Design review of the part built by this model. Coordinates are the model's own, in mm. A direction names the side the tool comes from. Give positions to 0.01 mm unless a question says otherwise; leave off trailing zeros. Order: outer loops, then holes, each group sorted by start corner. A loop starts at its lowest first (then second) coordinate and runs counter-clockwise, first axis right, second up.
```python
from build123d import *

# Parameters (mm, degrees)
SKETCH1_W           = 83
SKETCH1_H           = 151.45
BOSS_EXTRUDE1_DEPTH = 3
SKETCH2_W           = 83
SKETCH2_H           = 70
BOSS_EXTRUDE2_DEPTH = 3
SKETCH3_W           = 83
SKETCH3_H           = 89
BOSS_EXTRUDE3_DEPTH = 3
SKETCH6_W           = 34
SKETCH6_H           = 28
SKETCH6_R           = 4.15
SKETCH6_H_2         = 30
BOSS_EXTRUDE6_DEPTH = 30
SKETCH7_R           = 16
SKETCH7_R_2         = 15
BOSS_EXTRUDE7_DEPTH = 42
SKETCH8_R           = 5
CUT_EXTRUDE1_DEPTH  = 20.05


with BuildPart() as part:
    # Sketch1 → Boss-Extrude1 (new body)
    with BuildSketch(Plane.XY):
        with Locations((41.5, 75.725)):
            Rectangle(SKETCH1_W, SKETCH1_H)
    extrude(amount=BOSS_EXTRUDE1_DEPTH)

    # Sketch2 → Boss-Extrude2 (add)
    with BuildSketch(Plane(origin=(0, 16.05, 0), x_dir=(-1, 0, 0), z_dir=(0, -1, 0))):
        with Locations((-41.5, -38)):
            Rectangle(SKETCH2_W, SKETCH2_H)
    boss_extrude2 = extrude(amount=-BOSS_EXTRUDE2_DEPTH)

    # Mirror1: Boss-Extrude2 across plane
    add(boss_extrude2.mirror(Plane.ZX.offset(75.725)))

    # Sketch3 → Boss-Extrude3 (add)
    with BuildSketch(Plane(origin=(0, 135.4, 0), x_dir=(1, 0, 0), z_dir=(0, 1, 0))):
        with Locations((41.5, -47.5)):
            Rectangle(SKETCH3_W, SKETCH3_H)
    extrude(amount=-BOSS_EXTRUDE3_DEPTH)

    # Sketch6 → Boss-Extrude6 (add)
    with BuildSketch(Plane(origin=(0, 88.45, 0), x_dir=(1, 0, 0), z_dir=(0, 1, 0))):
        with Locations((21.979, 14)):
            Rectangle(SKETCH6_W, SKETCH6_H)
        with Locations((21.979, 18)):
            Circle(SKETCH6_R, mode=Mode.SUBTRACT)
        with Locations((60.98, 15)):
            Rectangle(SKETCH6_W, SKETCH6_H_2)
        with Locations((60.98, 18)):
            Circle(SKETCH6_R, mode=Mode.SUBTRACT)
    extrude(amount=-BOSS_EXTRUDE6_DEPTH)

    # Sketch7 → Boss-Extrude7 (add)
    with BuildSketch(Plane.XZ.offset(-132.4)):
        with Locations((42, 43)):
            Circle(SKETCH7_R)
        with Locations((42, 43)):
            Circle(SKETCH7_R_2, mode=Mode.SUBTRACT)
    extrude(amount=BOSS_EXTRUDE7_DEPTH)

    # Sketch8 → Cut-Extrude1 (cut, through all)
    with BuildSketch(Plane(origin=(0, 19.05, 0), x_dir=(1, 0, 0), z_dir=(0, 1, 0))):
        with Locations((42, -43)):
            Circle(SKETCH8_R)
    extrude(amount=-CUT_EXTRUDE1_DEPTH, mode=Mode.SUBTRACT)


solid = part.part
```
1. For pin 1 (8.5 mm diameter, centred on y = 79, z = -15.5, fed in from -X); pin 2 (1.5 mm diameter, centred on x = 44, y = 21.5, fed in from +Z); pin 3 (9 mm diameter, centred on x = 63.5, z = -21, fed in from +Y), all flat-tipped, find the tip position at first contact; note any pin that passes through.
Recorded:
pin 1: stops at x = 4.98
pin 2: stops at z = 3
pin 3: stops at y = 88.45
2. Take a section at B-B (y = 94.5). State the section outline as (x, z) points.
Recorded:
outline: (0, 0) - (83, 0) - (83, 3) - (0, 3) - close; circle Ø32 at (42, 43); hole circle Ø30 at (42, 43)
3. For line 1 along Z through (x, y) = (42, 99); line 2 along X through (y, z) = (67, -18); line 3 along Y through (x, z) = (22, 8.5), list the stretches that pass through material, from the lowest coordinate up.
Recorded:
line 1: z = 0 to 3, 27 to 28, 58 to 59
line 2: x = 4.98 to 17.83, 26.13 to 38.98, 43.98 to 56.83, 65.13 to 77.98
line 3: y = 16.05 to 19.05, 132.4 to 135.4
4. Take a section at C-C (x = 42). State the section outline as (y, z) points, then the cut area to 3 significant figures.
Recorded:
outline: (0, 0) - (151.45, 0) - (151.45, 3) - (135.4, 3) - (135.4, 92) - (132.4, 92) - (132.4, 59) - (90.4, 59) - (90.4, 58) - (132.4, 58) - (132.4, 28) - (90.4, 28) - (90.4, 27) - (132.4, 27) - (132.4, 3) - (19.05, 3) - (19.05, 38) - (16.05, 38) - (16.05, 3) - (0, 3) - close; (16.05, 48) - (19.05, 48) - (19.05, 73) - (16.05, 73) - close
area: 985 mm2
5. Take a section at D-D (z = 6.5). State the section outline as (x, y) points.
Recorded:
outline: (0, 16.05) - (83, 16.05) - (83, 19.05) - (0, 19.05) - close; (0, 132.4) - (83, 132.4) - (83, 135.4) - (0, 135.4) - close
6. Take a section at A-A (z = -18). State the section outline as (x, y) points.
Recorded:
outline: (4.98, 58.45) - (17.83, 58.45) - (17.83, 88.45) - (4.98, 88.45) - close; (26.13, 58.45) - (38.98, 58.45) - (38.98, 88.45) - (26.13, 88.45) - close; (43.98, 58.45) - (56.83, 58.45) - (56.83, 88.45) - (43.98, 88.45) - close; (65.13, 58.45) - (77.98, 58.45) - (77.98, 88.45) - (65.13, 88.45) - close
7. Draft analysis for pull direction Z (two halves, no side actions). For faces 1 (the face through (23.894, 73.66, -14.318)), 2 (the face through (41, 144, 3)), 3 (the face through (22, 58.45, -11)), state which applies: pulls with the +Z half, pulls with the -Z half, needs draft (parallel to the pull), parting line crosses it, or undercut.
Recorded:
face 1: undercut
face 2: pulls with the +Z half
face 3: needs draft
8. Machinability: for faces 4 (the face through (22, 88.45, -11)), 5 (the face through (42.1, 19.05, 37.5)), 6 (the face through (42.1, 16.05, 37.5)), 7 (the face through (77.98, 74, -15)), which of the approach directions +Z, -Z, +X, -X, +Y, -Y give a long, thin tool a straight path to every point of the face, cutting with its end or side? Answer none if there is none.
Recorded:
face 4: -Z, +X, -X, +Y
face 5: +Z, +X, -X
face 6: +Z, +X, -X, -Y
face 7: -Z, +X, +Y, -Y
